```python
from build123d import *


with BuildPart() as part:
    # Esquisse1 → Révolution1 (revolve)
    with BuildSketch(Plane.XY, mode=Mode.PRIVATE) as r_volution1_sk:
        with BuildLine():
            Line((-5.95, 2), (-5.55, 2))
            ThreePointArc((-5.55, 2), (-4.984314575, 1.765685425), (-4.75, 1.2))
            Line((-4.75, 1.2), (-4.75, 0.8))
            ThreePointArc((-4.75, 0.8), (-4.984314575, 0.234314575), (-5.55, 0))
            Line((-5.55, 0), (-5.95, 0))
            ThreePointArc((-5.95, 0), (-6.515685425, 0.234314575), (-6.75, 0.8))
            Line((-6.75, 0.8), (-6.75, 1.2))
            ThreePointArc((-6.75, 1.2), (-6.515685425, 1.765685425), (-5.95, 2))
        make_face()
    revolve(r_volution1_sk.sketch.rotate(Axis((0, 0, 0), (0, 1, 0)), 270), axis=Axis((0, 0, 0), (0, 1, 0)))


solid = part.part
```
For this review, take the finished solid that the model builds, in its own axes (mm). Coordinates: 2 decimals unless noted, no trailing zeros. Write each loop counter-clockwise with the first axis right and the second up, starting at its lowest first coordinate (ties: lowest second). Pieces come first, ordered by that corner, then holes.
(1) Add section D-D on y = 0.2. Give the boundary of the cut face in (x, z), then the cut area to 3 significant figures.
(2) Add section B-B on x = 0. Give the boundary of the cut face in (y, z), then the cut area to 3 significant figures.
(3) For pin 1 Ø1 at (x, y) = (-1.5, 1) entering from +Z, flat-tipped, find the tip position at first contact; note if it passes through.
(4) Add section C-C on y = 1. Give the boundary of the cut face in (x, z).
(5) Add section A-A on z = 0. Give the boundary of the cut face in (x, y), then the cut area to 3 significant figures.
(6) The part is to be moulded in two halves that separate along Z. For faces 1 (the face through (2.89, 1, 3.77)), 2 (the face through (6.59, 1, 1.46)), say which applies: +Z half, -Z half, draft (parallel to the pull), parting line (faces both ways), or undercut.
(7) Wall thickness on probe 1 along X at (y, z) = (0.95, 0); probe 2 along X at (y, z) = (1.25, -4.25); probe 3 along Z at (x, y) = (3, 0.8): over which ranges is each line inside the solid? List them lowest first.
Answer sheet:
1. outline: circle Ø12.96 at (0, 0); hole circle Ø10.04 at (0, 0)
1. area: 52.7 mm2
2. outline: (0, -5.95) arc R0.8 ccw to (0.8, -6.75) - (1.2, -6.75) arc R0.8 ccw to (2, -5.95) - (2, -5.55) arc R0.8 ccw to (1.2, -4.75) - (0.8, -4.75) arc R0.8 ccw to (0, -5.55) - close; (0, 5.55) arc R0.8 ccw to (0.8, 4.75) - (1.2, 4.75) arc R0.8 ccw to (2, 5.55) - (2, 5.95) arc R0.8 ccw to (1.2, 6.75) - (0.8, 6.75) arc R0.8 ccw to (0, 5.95) - close
2. area: 6.90 mm2
3. pin 1: stops at z = 6.68
4. outline: circle Ø13.5 at (0, 0); hole circle Ø9.5 at (0, 0)
5. outline: (-6.75, 0.8) arc R0.8 ccw to (-5.95, 0) - (-5.55, 0) arc R0.8 ccw to (-4.75, 0.8) - (-4.75, 1.2) arc R0.8 ccw to (-5.55, 2) - (-5.95, 2) arc R0.8 ccw to (-6.75, 1.2) - close; (4.75, 0.8) arc R0.8 ccw to (5.55, 0) - (5.95, 0) arc R0.8 ccw to (6.75, 0.8) - (6.75, 1.2) arc R0.8 ccw to (5.95, 2) - (5.55, 2) arc R0.8 ccw to (4.75, 1.2) - close
5. area: 6.90 mm2
6. face 1: undercut
6. face 2: parting line
7. probe 1: x = -6.75 to -4.75, 4.75 to 6.75
7. probe 2: x = -5.24 to -2.12, 2.12 to 5.24
7. probe 3: z = -6.05 to -3.68, 3.68 to 6.05
